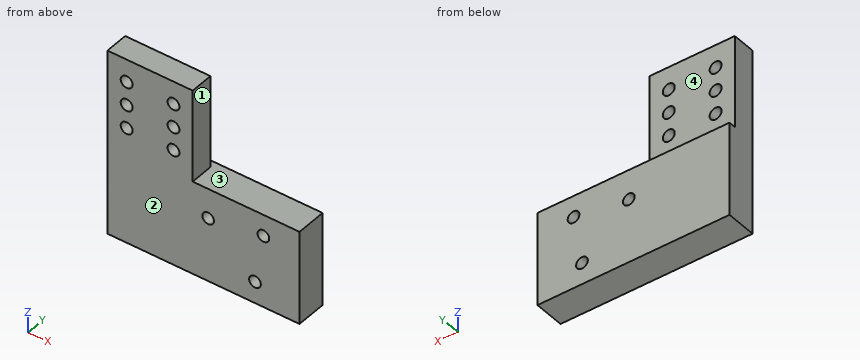
```python
from build123d import *

# Parameters (mm, degrees)
SKETCH1_W                = 36.4
SKETCH1_H                = 39.5
SKETCH1_R                = 2.55
BOSS_EXTRUDE1_DEPTH      = 10
BOSS_EXTRUDE2_DEPTH      = 3
BOSS_EXTRUDE2_DEPTH_BACK = 10
SKETCH2_W                = 82
SKETCH2_H                = 40
F_5_0MM_DOWEL_HOLE1_D    = 5


with BuildPart() as part:
    # Sketch1 → Boss-Extrude1 (new body)
    with BuildSketch(Plane(origin=(0, 0, 0), x_dir=(1, 0, 0), z_dir=(0, 1, 0))):
        with Locations((18.2, 19.75)):
            Rectangle(SKETCH1_W, SKETCH1_H)
        with Locations(Location((8.2, 29.75, 0), (0, 0, 270))):
            Circle(SKETCH1_R, mode=Mode.SUBTRACT)
        with Locations(Location((28.2, 29.75, 0), (0, 0, 270))):
            Circle(SKETCH1_R, mode=Mode.SUBTRACT)
        with Locations(Location((28.2, 19.75, 0), (0, 0, 270))):
            Circle(SKETCH1_R, mode=Mode.SUBTRACT)
        with Locations(Location((28.2, 9.75, 0), (0, 0, 270))):
            Circle(SKETCH1_R, mode=Mode.SUBTRACT)
        with Locations(Location((8.2, 19.75, 0), (0, 0, 270))):
            Circle(SKETCH1_R, mode=Mode.SUBTRACT)
        with Locations(Location((8.2, 9.75, 0), (0, 0, 270))):
            Circle(SKETCH1_R, mode=Mode.SUBTRACT)
    extrude(amount=BOSS_EXTRUDE1_DEPTH)

    # Sketch2 → Boss-Extrude2 (add, two sides: drawn at the far end of the back side and taken through both)
    with BuildSketch(Plane(origin=(0, 10, 0), x_dir=(1, 0, 0), z_dir=(0, 1, 0)).offset(-BOSS_EXTRUDE2_DEPTH_BACK)):
        with Locations((41, 59.5)):
            Rectangle(SKETCH2_W, SKETCH2_H)
    extrude(amount=BOSS_EXTRUDE2_DEPTH + BOSS_EXTRUDE2_DEPTH_BACK)

    # Ø5.0mm Dowel Hole1 (through all)
    with Locations(Plane(origin=(42.996100309, 13, -52.245667008), x_dir=(0, 0, 1), z_dir=(0, 1, 0))):
        with Locations((0, 0), (-18, 20), (3.585786438, 23.585786437)):
            Hole(F_5_0MM_DOWEL_HOLE1_D / 2)


solid = part.part
```
Can you work these out from the model? Positions are in its coordinate system, mm. Face numbers are marked on the shaded views. A direction names the side the tool comes from. Round coordinates to 2 decimals unless told otherwise and drop trailing zeros. Loops run counter-clockwise (first coordinate to the right, second up) from the corner with the lowest first, then second, coordinate; pieces in that order, holes last. Notation, with made-up numbers: M 47.25,83.25 L 60.25,83.25 A32 cw 60.25,114.25 Z; hole C -21.5,47 d3. An arc over 180 degrees is marked long. Answer as a JSON object with one key per item and string values. Group by question number.
Q1. Imagine slicing it at C-C, the plane y = 9. Count the separate pieces of the cut face and the enclosed holes in it, then the cut area to 3 significant figures.
Q2. Imagine slicing it at D-D, the plane x = 12. Please give me the cut outline in (y, z), then the cut area to 3 significant figures.
Q3. Imagine slicing it at B-B, the plane x = 28.2. Please give me the cut outline in (y, z).
Q4. Imagine slicing it at A-A, the plane z = -9.75. Please give me the cut outline in (x, y), then the cut area to 3 significant figures.
Q5. Please list where these lines run through material, in increasing order: L1, parallel to X at y = 8.25, z = -29.75; L2, parallel to Z at x = 28.5, y = 1.75; L3, parallel to X at y = 3, z = -8.
Q6. On a 3-axis mill with a long thin cutter (end or side, diameter ignored), from which of +Z, -Z, +X, -X, +Y, -Y can I reach the whole of each face in a straight line? I mean the marked faces 1, 2, 3 and 4. Say none if no direction works.
Q7. Will these pins go through, and if not, where does the flat tip stop? pin 1 (6.5 mm diameter, centred on x = 8.2, z = -29.75, fed in from +Y); pin 2 (3 mm diameter, centred on y = 3, z = -34, fed in from +X); pin 3 (2 mm diameter, centred on x = 48.5, y = 11, fed in from +Z).
Findings:
{
 "1": {"separate pieces": "1", "enclosed holes": "9", "area": "4,540 mm2"},
 "2": {"outline": "M 0,-79.5 L 13,-79.5 L 13,-39.5 L 10,-39.5 L 10,0 L 0,0 Z", "area": "915 mm2"},
 "3": {"outline": "M 0,-79.5 L 13,-79.5 L 13,-39.5 L 10,-39.5 L 10,-32.3 L 0,-32.3 Z; M 0,-27.2 L 10,-27.2 L 10,-22.3 L 0,-22.3 Z; M 0,-17.2 L 10,-17.2 L 10,-12.3 L 0,-12.3 Z; M 0,-7.2 L 10,-7.2 L 10,0 L 0,0 Z"},
 "4": {"outline": "M 0,0 L 5.65,0 L 5.65,10 L 0,10 Z; M 10.75,0 L 25.65,0 L 25.65,10 L 10.75,10 Z; M 30.75,0 L 36.4,0 L 36.4,10 L 30.75,10 Z", "area": "262 mm2"},
 "5": {"L1": "x = 0 to 5.65, 10.75 to 25.65, 30.75 to 36.4", "L2": "z = -79.5 to -32.28, -27.22 to -22.28, -17.22 to -12.28, -7.22 to 0", "L3": "x = 0 to 6.35, 10.05 to 26.35, 30.05 to 36.4"},
 "6": {"face 1": "+Z, +X, +Y, -Y", "face 2": "+Z, -Z, +X, -X, -Y", "face 3": "+Z, +X, +Y", "face 4": "+Z, +X, -X, +Y"},
 "7": {"pin 1": "stops at y = 10", "pin 2": "stops at x = 36.4", "pin 3": "stops at z = -39.5"}
}
